```python
from build123d import *

# Parameters (mm, degrees)
SKETCH_1_W          = 140
SKETCH_1_H          = 20
SKETCH_1_R          = 1.9
EXTRUDE_1_DEPTH     = 10
SKETCH_2_W          = 65
SKETCH_2_H          = 6
EXTRUDE_2_DEPTH     = 140
SKETCH_3_R          = 1.9
CUT_EXTRUDE_1_DEPTH = 10


with BuildPart() as part:
    # 草图1 → 凸台-拉伸1 (new body)
    with BuildSketch(Plane.XY):
        with Locations((70, -10)):
            Rectangle(SKETCH_1_W, SKETCH_1_H)
        with Locations((10, -10)):
            Circle(SKETCH_1_R, mode=Mode.SUBTRACT)
        with Locations((40, -10)):
            Circle(SKETCH_1_R, mode=Mode.SUBTRACT)
        with Locations((70, -10)):
            Circle(SKETCH_1_R, mode=Mode.SUBTRACT)
        with Locations((100, -10)):
            Circle(SKETCH_1_R, mode=Mode.SUBTRACT)
        with Locations((130, -10)):
            Circle(SKETCH_1_R, mode=Mode.SUBTRACT)
    extrude(amount=EXTRUDE_1_DEPTH)

    # 草图2 → 凸台-拉伸2 (add, through all)
    with BuildSketch(Plane.ZY):
        with Locations((-22.5, -3)):
            Rectangle(SKETCH_2_W, SKETCH_2_H)
    extrude(amount=-EXTRUDE_2_DEPTH)

    # 草图3 → 切除-拉伸1 (cut)
    with BuildSketch(Plane.XZ.offset(6)):
        with BuildLine():
            ThreePointArc((44.9, -35), (43, -33.1), (41.1, -35))
            Line((41.1, -35), (43, -35))
            Line((43, -35), (43, -36.9))
            ThreePointArc((43, -36.9), (44.343502884, -36.343502884), (44.9, -35))
        make_face()
        with BuildLine():
            Line((43, -35), (41.1, -35))
            ThreePointArc((41.1, -35), (41.656497116, -36.343502884), (43, -36.9))
            Line((43, -36.9), (43, -35))
        make_face()
        with BuildLine():
            ThreePointArc((44.9, -50), (44.343502884, -48.656497116), (43, -48.1))
            Line((43, -48.1), (43, -50))
            Line((43, -50), (41.1, -50))
            ThreePointArc((41.1, -50), (43, -51.9), (44.9, -50))
        make_face()
        with BuildLine():
            Line((43, -50), (43, -48.1))
            ThreePointArc((43, -48.1), (41.656497116, -48.656497116), (41.1, -50))
            Line((41.1, -50), (43, -50))
        make_face()
        with BuildLine():
            ThreePointArc((16.9, -50), (16.343502884, -48.656497116), (15, -48.1))
            Line((15, -48.1), (15, -50))
            Line((15, -50), (16.9, -50))
        make_face()
        with BuildLine():
            Line((15, -50), (15, -48.1))
            ThreePointArc((15, -48.1), (13.656497116, -51.343502884), (16.9, -50))
            Line((16.9, -50), (15, -50))
        make_face()
        with BuildLine():
            Line((15, -36.9), (15, -35))
            Line((15, -35), (16.9, -35))
            ThreePointArc((16.9, -35), (13.656497116, -33.656497116), (15, -36.9))
        make_face()
        with BuildLine():
            Line((16.9, -35), (15, -35))
            Line((15, -35), (15, -36.9))
            ThreePointArc((15, -36.9), (16.343502884, -36.343502884), (16.9, -35))
        make_face()
        with Locations(Location((15, -10, 0), (0, 0, 270))):
            Circle(SKETCH_3_R)
        with Locations(Location((15, -25, 0), (0, 0, 270))):
            Circle(SKETCH_3_R)
        with Locations(Location((43, -25, 0), (0, 0, 270))):
            Circle(SKETCH_3_R)
        with Locations(Location((43, -10, 0), (0, 0, 270))):
            Circle(SKETCH_3_R)
        with Locations(Location((97, -10, 0), (0, 0, 270))):
            Circle(SKETCH_3_R)
        with Locations(Location((97, -35, 0), (0, 0, 270))):
            Circle(SKETCH_3_R)
        with Locations(Location((97, -50, 0), (0, 0, 270))):
            Circle(SKETCH_3_R)
        with Locations(Location((125, -50, 0), (0, 0, 270))):
            Circle(SKETCH_3_R)
        with Locations(Location((125, -35, 0), (0, 0, 270))):
            Circle(SKETCH_3_R)
        with Locations(Location((125, -25, 0), (0, 0, 270))):
            Circle(SKETCH_3_R)
        with Locations(Location((125, -10, 0), (0, 0, 270))):
            Circle(SKETCH_3_R)
        with Locations(Location((97, -25, 0), (0, 0, 270))):
            Circle(SKETCH_3_R)
    extrude(amount=-CUT_EXTRUDE_1_DEPTH, mode=Mode.SUBTRACT)


solid = part.part
```
Verification items for the finished model (mm, model axes). A direction names the side the tool comes from. Coordinates: 2 decimals unless noted, no trailing zeros. Loops run counter-clockwise (first coordinate to the right, second up) from the corner with the lowest first, then second, coordinate; pieces in that order, holes last. Notation, with made-up numbers: (53, -18.75) - (81, -18.75) arc R22 ccw to (81, 11.25) - close; hole circle Ø9 at (61.25, 85). An arc over 180 degrees is marked (long way). Answer as a JSON object with one key per item and string values.
(1) Scan lines: line 1 along X through (y, z) = (-2.65, -10); line 2 along Y through (x, z) = (40, 3.5); line 3 along Y through (x, z) = (66.5, -11). Record each from-to range of solid material in increasing order.
Response:
{"line 1": "x = 0 to 13.1, 16.9 to 41.1, 44.9 to 95.1, 98.9 to 123.1, 126.9 to 140", "line 2": "y = -20 to -11.9, -8.1 to 0", "line 3": "y = -6 to 0"}
(2) Go/stop test with flat-tipped pins: pin 1 Ø1 at (x, z) = (118, -40.5) entering from +Y; pin 2 Ø2.5 at (x, y) = (130, -10) entering from -Z; pin 3 Ø4.5 at (x, z) = (15, -50) entering from -Y; pin 4 Ø12 at (x, y) = (58.5, -17.5) entering from -Z. Record where each tip stops, or that it passes through.
Response:
{"pin 1": "stops at y = 0", "pin 2": "passes through", "pin 3": "stops at y = -6", "pin 4": "stops at z = 0"}
(3) Mould release check, pull along Y, two halves, no side actions. Record for faces 1 (the flat face through (69, -20, 5)), 2 (the cylindrical face through (10.877, -11.686, 4.93)), 3 (the cylindrical face through (68.492, -11.156, 4.93)), 4 (the cylindrical face through (41.314, -3.042, -10.877)): pulls with the +Y half, pulls with the -Y half, needs draft (parallel to the pull), parting line crosses it, or undercut.
Response:
{"face 1": "pulls with the -Y half", "face 2": "undercut", "face 3": "undercut", "face 4": "needs draft"}
(4) Access from +Z, -Z, +X, -X, +Y, -Y to the whole of each face (thin tool, end or side, straight path). Record for faces 5 (the flat face through (69, -13, 0)), 6 (the cylindrical face through (98.1, -9.92, 4.93)).
Response:
{"face 5": "-Z, +X, -X, -Y", "face 6": "+Z, -Z"}
(5) Cross-section at D-D, the plane z = 3. Record the boundary of the cut face in (x, y), then the cut area to 3 significant figures.
Response:
{"outline": "(0, -20) - (140, -20) - (140, 0) - (0, 0) - close; hole circle Ø3.8 at (10, -10); hole circle Ø3.8 at (40, -10); hole circle Ø3.8 at (70, -10); hole circle Ø3.8 at (100, -10); hole circle Ø3.8 at (130, -10)", "area": "2,740 mm²"}
(6) Cross-section at C-C, the plane z = -25. Record the boundary of the cut face in (x, y), then the cut area to 3 significant figures.
Response:
{"outline": "(0, -6) - (13.1, -6) - (13.1, 0) - (0, 0) - close; (16.9, -6) - (41.1, -6) - (41.1, 0) - (16.9, 0) - close; (44.9, -6) - (95.1, -6) - (95.1, 0) - (44.9, 0) - close; (98.9, -6) - (123.1, -6) - (123.1, 0) - (98.9, 0) - close; (126.9, -6) - (140, -6) - (140, 0) - (126.9, 0) - close", "area": "749 mm²"}
(7) Cross-section at A-A, the plane x = 10. Record the boundary of the cut face in (y, z).
Response:
{"outline": "(-20, 0) - (-11.9, 0) - (-11.9, 10) - (-20, 10) - close; (-8.1, 0) - (-6, 0) - (-6, -55) - (0, -55) - (0, 10) - (-8.1, 10) - close"}
(8) Cross-section at B-B, the plane y = -3. Count the separate pieces of the cut face and the enclosed holes in it, then the cut area to 3 significant figures.
Response:
{"separate pieces": "1", "enclosed holes": "16", "area": "8,920 mm²"}
